Here's the drawing with two shaded views (mm, measured from the low corner). I have some questions. A direction names the side the tool comes from. Round coordinates to 2 decimals unless told otherwise and drop trailing zeros. Loops run counter-clockwise (first coordinate to the right, second up) from the corner with the lowest first, then second, coordinate; pieces in that order, holes last. Notation, with made-up numbers: (-22, -3.75) -> (-11, -3.75) arc R26 ccw to (-11, 35.25) -> close; hole circle Ø7 at (51, 28.25). An arc over 180 degrees is marked (long way). Write each question's results on one line, items separated by ' | '.
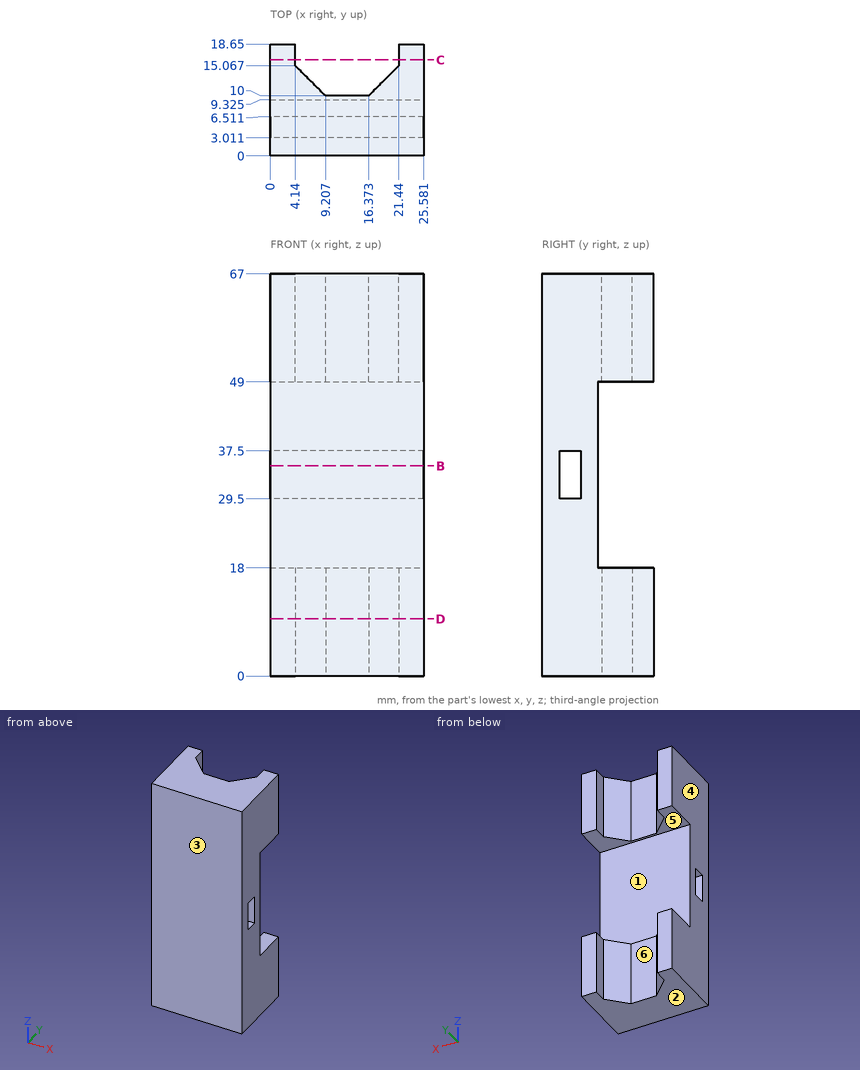
1. If we section it at B-B (z = 35): List the corners of the cut face in (x, y) for me (1 decimal).
Final values:
outline: (0, 0) -> (25.6, 0) -> (25.6, 3) -> (0, 3) -> close; (0, 6.5) -> (25.6, 6.5) -> (25.6, 9.3) -> (0, 9.3) -> close
2. Will these pins go through, and if not, where does the flat tip stop? pin 1 (4 mm diameter, centred on x = 6.5, z = 35.5, fed in from +Y) (1 decimal); pin 2 (2 mm diameter, centred on x = 13.5, z = 58, fed in from +Y); pin 3 (6 mm diameter, centred on x = 17, z = 15, fed in from +Y) (1 decimal).
Final values:
pin 1: y = 9.3 | pin 2: y = 10 | pin 3: y = 13.6
3. On a 3-axis mill with a long thin cutter (end or side, diameter ignored), from which of +Z, -Z, +X, -X, +Y, -Y can I reach the whole of each face in a straight line? I mean the marked faces 4, 5 and 6. Say none if no direction works.
Final values:
face 4: +Z, -Z, -X, +Y, -Y | face 5: +X, -X, +Y | face 6: +Z, -Z, +Y
4. Please list where these lines run through material, in increasing order: line 1 (Z direction, x = 2.25, y = 4.5); line 2 (X direction, y = 16.5, z = 8.5); line 3 (Y direction, x = 18, z = 35) (1 decimal). Write a range as from..to.
Final values:
line 1: 0..29.5, 37.5..67 | line 2: 0..4.14, 21.44..25.58 | line 3: 0..3, 6.5..9.3
5. We'd pull the mould along Z, two halves only. Please class the marked faces 1, 2 and 3: pulls with the +Z half, pulls with the -Z half, needs draft (parallel to the pull), parting line crosses it, or undercut.
Final values:
face 1: undercut | face 2: pulls with the -Z half | face 3: needs draft
6. If we section it at D-D (z = 9.5): List the corners of the cut face in (x, y) for me, then the cut area to 3 significant figures.
Final values:
outline: (0, 0) -> (25.58, 0) -> (25.58, 18.65) -> (21.44, 18.65) -> (21.44, 15.07) -> (16.37, 10) -> (9.21, 10) -> (4.14, 15.07) -> (4.14, 18.65) -> (0, 18.65) -> close | area: 353 mm2
7. If we section it at C-C (y = 16): List the corners of the cut face in (x, z) for me, then the cut area to 3 significant figures.
Final values:
outline: (0, 0) -> (4.14, 0) -> (4.14, 18) -> (0, 18) -> close; (0, 49) -> (4.14, 49) -> (4.14, 67) -> (0, 67) -> close; (21.44, 0) -> (25.58, 0) -> (25.58, 18) -> (21.44, 18) -> close; (21.44, 49) -> (25.58, 49) -> (25.58, 67) -> (21.44, 67) -> close | area: 298 mm2
